The model under review builds one solid part; all positions refer to its coordinate system, in mm. Face numbers are marked on the shaded views. A direction names the side the tool comes from. Coordinates: 2 decimals unless noted, no trailing zeros. Write each loop counter-clockwise with the first axis right and the second up, starting at its lowest first coordinate (ties: lowest second). Pieces come first, ordered by that corner, then holes. Notation, with made-up numbers: (-31, 65.5) -> (23, 65.5) arc R10 ccw to (23, 74.5) -> close; hole circle Ø3 at (84, 39). An arc over 180 degrees is marked (long way). Put each result on its own line as item: value. Start each with the question number.
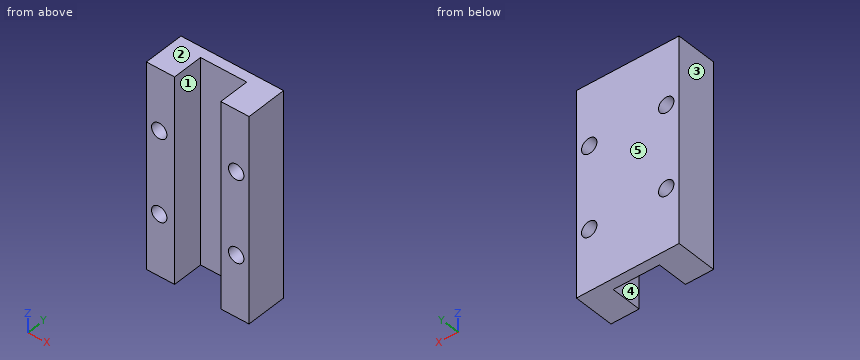
from build123d import *

# Parameters (mm, degrees)
SKETCH_1_W          = 20
SKETCH_1_H          = 39.9
SKETCH_1_R          = 1.5
EXTRUDE_1_DEPTH     = 8
SKETCH_2_W          = 9
SKETCH_2_H          = 6
CUT_EXTRUDE_1_DEPTH = 60


with BuildPart() as part:
    # 草图1 → 凸台-拉伸1 (new body)
    with BuildSketch(Plane(origin=(0, 0, 0), x_dir=(1, 0, 0), z_dir=(0, 1, 0))):
        Rectangle(SKETCH_1_W, SKETCH_1_H)
        with Locations(Location((-7.5, 8, 0), (0, 0, 270))):
            Circle(SKETCH_1_R, mode=Mode.SUBTRACT)
        with Locations(Location((-7.5, -8, 0), (0, 0, 90))):
            Circle(SKETCH_1_R, mode=Mode.SUBTRACT)
        with Locations(Location((7.5, -8, 0), (0, 0, 270))):
            Circle(SKETCH_1_R, mode=Mode.SUBTRACT)
        with Locations(Location((7.5, 8, 0), (0, 0, 90))):
            Circle(SKETCH_1_R, mode=Mode.SUBTRACT)
    extrude(amount=EXTRUDE_1_DEPTH)

    # 草图2 → 切除-拉伸1 (cut)
    with BuildSketch(Plane.XY.offset(19.95)):
        with Locations((0, 3)):
            Rectangle(SKETCH_2_W, SKETCH_2_H)
    extrude(amount=-CUT_EXTRUDE_1_DEPTH, mode=Mode.SUBTRACT)


solid = part.part
1. Consider section D-D on y = 6.75. State the section outline as (x, z) points.
2. The part is to be moulded in two halves that separate along X. For the marked faces 1, 2 and 3, say which applies: released by +X, released by -X, zero draft, split by the parting line, or undercut.
3. Consider section B-B on z = 8. State the section outline as (x, y) points, then the cut area to 3 significant figures.
4. Insertion check: P1, Ø2.5, axis at x = 7.5, z = -8, coming from the -Y side; P2, Ø7, axis at x = -0.5, z = -4, coming from the -Y side. Each pin has a flat end and moves straight along its axis. Give the tip position at first contact, or say it passes through.
5. Tool access review of the marked faces 4 and 5: name each direction out of +Z, -Z, +X, -X, +Y, -Y from which nothing blocks a thin tool from reaching the whole face with its end or side.
6. Consider section C-C on x = 7.5. State the section outline as (y, z) points, then the cut area to 3 significant figures.
7. Consider section A-A on y = 2.25. State the section outline as (x, z) points, then the cut area to 3 significant figures.
8. Wall thickness on line 1 (X direction, y = 4.5, z = -8); line 2 (X direction, y = 3, z = 17.5); line 3 (Z direction, x = 6.75, y = 4.25): over which ranges is each line inside the solid? List them lowest first. Write a range as from..to.
Output values:
1. outline: (-10, -19.95) -> (10, -19.95) -> (10, 19.95) -> (-10, 19.95) -> close; hole circle Ø3 at (-7.5, -8); hole circle Ø3 at (-7.5, 8); hole circle Ø3 at (7.5, -8); hole circle Ø3 at (7.5, 8)
2. face 1: undercut
2. face 2: zero draft
2. face 3: released by -X
3. outline: (-10, 0) -> (-9, 0) -> (-9, 8) -> (-10, 8) -> close; (-6, 0) -> (-4.5, 0) -> (-4.5, 6) -> (4.5, 6) -> (4.5, 0) -> (6, 0) -> (6, 8) -> (-6, 8) -> close; (9, 0) -> (10, 0) -> (10, 8) -> (9, 8) -> close
3. area: 58.0 mm^2
4. P1: passes through
4. P2: stops at y = 6
5. face 4: +Z, -Z, -Y
5. face 5: +Z, -Z, +X, -X, +Y
6. outline: (0, -19.95) -> (8, -19.95) -> (8, -9.5) -> (0, -9.5) -> close; (0, -6.5) -> (8, -6.5) -> (8, 6.5) -> (0, 6.5) -> close; (0, 9.5) -> (8, 9.5) -> (8, 19.95) -> (0, 19.95) -> close
6. area: 271 mm^2
7. outline: (-10, -19.95) -> (-4.5, -19.95) -> (-4.5, 19.95) -> (-10, 19.95) -> close; (4.5, -19.95) -> (10, -19.95) -> (10, 19.95) -> (4.5, 19.95) -> close; hole circle Ø3 at (-7.5, -8); hole circle Ø3 at (-7.5, 8); hole circle Ø3 at (7.5, -8); hole circle Ø3 at (7.5, 8)
7. area: 411 mm^2
8. line 1: x = -10..-9, -6..-4.5, 4.5..6, 9..10
8. line 2: x = -10..-4.5, 4.5..10
8. line 3: z = -19.95..-9.3, -6.7..6.7, 9.3..19.95
